```python
from build123d import *

# Parameters (mm, degrees)
F1_DEPTH = 3.175
F2_R     = 0.635
F3_R     = 5.08


with BuildPart() as f1:
    # F0 (on Top) → F1 (new body)
    with BuildSketch(Plane.XY):
        Polygon((0, 5.08), (5.08, 0), (38.1, 0), (0, 38.1), align=None)
    extrude(amount=F1_DEPTH)

    # F2
    f2_edges = [f1.edges().sort_by_distance(p)[0] for p in [
        (0, 38.1, 1.5875),
        (38.1, 0, 1.5875),
    ]]
    fillet(f2_edges, radius=F2_R)

    # F3
    f3_edges = [f1.edges().sort_by_distance(p)[0] for p in [
        (5.08, 0, 1.5875),
        (0, 5.08, 1.5875),
    ]]
    fillet(f3_edges, radius=F3_R)


solid = f1.part
```
Build history of the part. All positions in model axes, mm. Coordinates: 2 decimals unless noted, no trailing zeros. Order: outer loops, then holes, each group sorted by start corner. A loop starts at its lowest first (then second) coordinate and runs counter-clockwise, first axis right, second up.
Item 1: Saw through at B-B on x = 16.5. List the corners of the cut face in (y, z) (3 decimals), then the cut area to 3 significant figures.
Filled in:
outline: (0, 0) - (21.6, 0) - (21.6, 3.175) - (0, 3.175) - close
area: 68.6 mm2
Item 2: Saw through at C-C on y = 23. List the corners of the cut face in (x, z) (3 decimals).
Filled in:
outline: (0, 0) - (15.1, 0) - (15.1, 3.175) - (0, 3.175) - close
Item 3: Saw through at A-A on z = 0.95. List the corners of the cut face in (x, y) (3 decimals).
Filled in:
outline: (0, 7.184) arc R5.08 ccw to (1.488, 3.592) - (3.592, 1.488) arc R5.08 ccw to (7.184, 0) - (36.567, 0) arc R0.635 ccw to (37.016, 1.084) - (1.084, 37.016) arc R0.635 ccw to (0, 36.567) - close
Item 4: Drill centre lines: L1, parallel to Y at x = 8, z = 1.1; L2, parallel to Y at x = 20, z = 2.1; L3, parallel to X at y = 11, z = 0.55. Where is each one in solid material? Low to high.
Filled in:
L1: y = 0 to 30.1
L2: y = 0 to 18.1
L3: x = 0 to 27.1
